The drawing under review shows one solid part. Ordinate dimensions are in mm from its lowest x, y, z. Give positions to 0.01 mm unless a question says otherwise; leave off trailing zeros. Loops run counter-clockwise (first coordinate to the right, second up) from the corner with the lowest first, then second, coordinate; pieces in that order, holes last. Notation, with made-up numbers: M 58.25,-33 L 72.25,-33 A33 cw 72.25,1 Z; hole C 60.25,72.5 d1. An arc over 180 degrees is marked long. One line per item, written item: value. Start each with the question number.
Q1. We need section B-B on x = 108. Write out the cut boundary in (y, z).
Q2. To check wall thickness, follow line 1 along Y through (x, z) = (96, 1.5) (1 decimal); line 2 along X through (y, z) = (60, 1.9) (1 decimal); line 3 along Y through (x, z) = (113, 0.95). State the ranges of each line that lie inside material, in increasing order. Write a range as from..to.
Q3. We need section C-C on y = 89. Write out the cut boundary in (x, z) (1 decimal).
Q4. We need section A-A on z = 1.1. Give the number of separate pieces and of enclosed holes in the cut face, plus the area to 3 significant figures.
Q5. For pin 1 (12 mm diameter, centred on x = 99.5, y = 70, fed in from -Z); pin 2 (1.6 mm diameter, centred on x = 45.71, y = 35.71, fed in from -Z), all flat-tipped, find the tip position at first contact; note any pin that passes through.
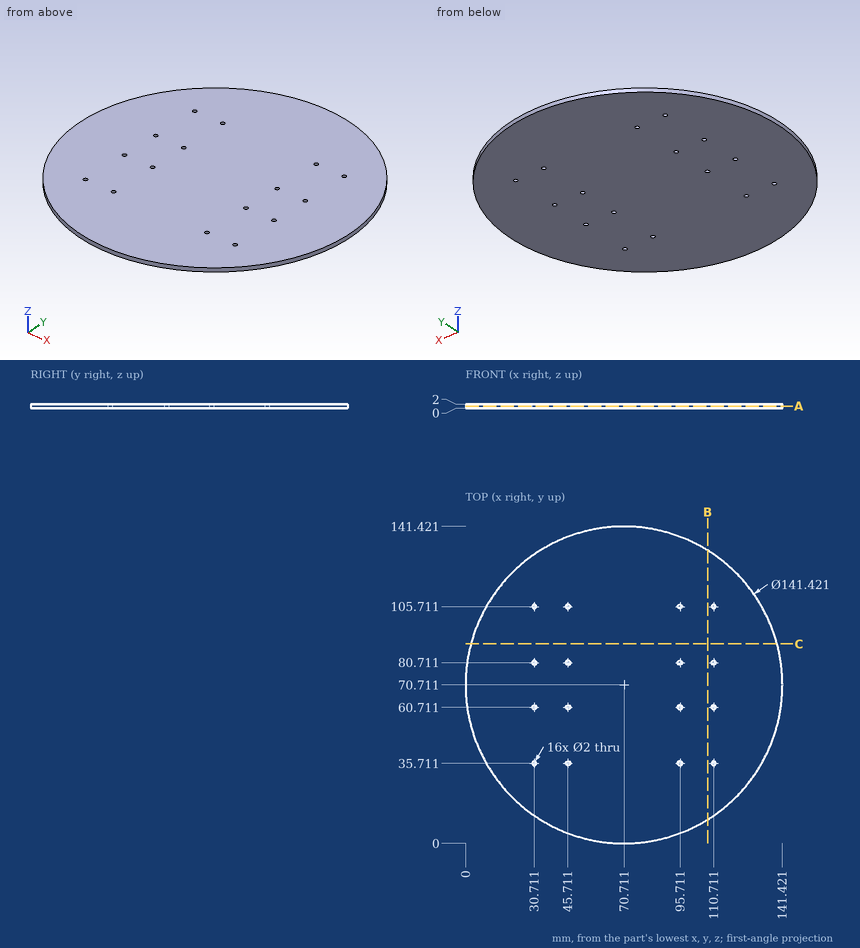
Solved:
1. outline: M 10.63,0 L 130.79,0 L 130.79,2 L 10.63,2 Z
2. line 1: 4.7..34.8, 36.7..59.8, 61.7..79.8, 81.7..104.8, 106.7..136.7
2. line 2: 0.8..30, 31.4..45, 46.4..95, 96.4..110, 111.4..140.6
2. line 3: 14.04..127.38
3. outline: M 2.4,0 L 139,0 L 139,2 L 2.4,2 Z
4. separate pieces: 1
4. enclosed holes: 16
4. area: 15,700 mm2
5. pin 1: z = 0
5. pin 2: through
